Can you work these out from the model? Positions are in its coordinate system, mm. A direction names the side the tool comes from. Coordinates: 2 decimals unless noted, no trailing zeros. Order: outer loops, then holes, each group sorted by start corner. A loop starts at its lowest first (then second) coordinate and runs counter-clockwise, first axis right, second up. Notation, with made-up numbers: (53, 49.25) -> (111, 49.25) arc R9 ccw to (111, 62.25) -> close; hole circle Ø9 at (72, -22.75). An arc over 180 degrees is marked (long way). Answer in a Markdown table with one row per item. Add a question column.
1. We'd pull the mould along X, two halves only. Please class faces 1 (the face through (7.938, 0, 5)), 2 (the face through (6.49, 0.01, -12.21)), 3 (the face through (0, -0.794, -7)), 4 (the face through (14.288, 0, 0)): pulls with the +X half, pulls with the -X half, needs draft (parallel to the pull), parting line crosses it, or undercut.
2. Imagine slicing it at B-B on z = 12.7. Write out the boundary of the cut face in (x, y) (1 decimal), plus the area to 3 significant figures.
3. Imagine slicing it at D-D on x = -8.75. Write out the boundary of the cut face in (y, z), plus the area to 3 significant figures.
4. Imagine slicing it at A-A on z = -5. Write out the boundary of the cut face in (x, y).
5. Will these pins go through, and if not, where does the flat tip stop? pin 1 (6 mm diameter, centred on x = -7.94, z = -10.32, fed in from -Y); pin 2 (0.8 mm diameter, centred on x = -3.5, y = 0, fed in from +Z); pin 3 (4 mm diameter, centred on x = -12.5, z = 13.5, fed in from +Y); pin 4 (2.5 mm diameter, centred on x = -11.11, z = 12.7, fed in from +Y).
6. If I drill on line 1 along X through (y, z) = (-0.3, 12.7) (1 decimal); line 2 along X through (y, z) = (-0.3, 6.5); line 3 along X through (y, z) = (0, -12), over which ranges is the centre line in solid material (lowest first)? Write a range as [from, to].
7. On a 3-axis mill with a long thin cutter (end or side, diameter ignored), from which of +Z, -Z, +X, -X, +Y, -Y can I reach the whole of each face in a straight line? I mean faces 5 (the face through (0, 0, -5.556)), 6 (the face through (-10, 0, 11)), 7 (the face through (0, 0, -15.081)). Say none if no direction works.
8. Imagine slicing it at C-C on y = 0.4. Write out the boundary of the cut face in (x, z), plus the area to 3 significant figures.
from build123d import *

# Parameters (mm, degrees)
BOSS_EXTRUDE1_DEPTH = 0.79375
SKETCH2_W           = 6.35
SKETCH2_H           = 4.7625
CUT_EXTRUDE1_DEPTH  = 0.79375
SKETCH3_R           = 1.5875
SKETCH3_R_2         = 2.38125
CUT_EXTRUDE2_DEPTH  = 1.5875


with BuildPart() as part:
    # Sketch1 → Boss-Extrude1 (new, symmetric)
    with BuildSketch(Plane(origin=(0, 0, 0), x_dir=(1, 0, 0), z_dir=(0, 1, 0))):
        Polygon((14.2875, 15.08125), (-14.2875, 15.08125), (-14.2875, -15.08125), (-7.9375, -15.08125), (-7.9375, 5.55625), (7.9375, 5.55625), (7.9375, -15.08125), (14.2875, -15.08125), align=None)
    extrude(amount=BOSS_EXTRUDE1_DEPTH, both=True)

    # Sketch2 → Cut-Extrude1 (cut)
    with BuildSketch(Plane(origin=(0, 0.79375, 0), x_dir=(1, 0, 0), z_dir=(0, 1, 0))):
        with Locations((-11.1125, -12.7)):
            Rectangle(SKETCH2_W, SKETCH2_H)
        with Locations((11.1125, -12.7)):
            Rectangle(SKETCH2_W, SKETCH2_H)
    extrude(amount=-CUT_EXTRUDE1_DEPTH, mode=Mode.SUBTRACT)

    # Sketch3 → Cut-Extrude2 (cut)
    with BuildSketch(Plane(origin=(0, 0.79375, 0), x_dir=(1, 0, 0), z_dir=(0, 1, 0))):
        with Locations(Location((-11.1125, -12.7, 0), (0, 0, 270))):
            Circle(SKETCH3_R)
        with Locations(Location((-7.9375, 10.31875, 0), (0, 0, 270))):
            Circle(SKETCH3_R_2)
        with Locations(Location((11.1125, -12.7, 0), (0, 0, 270))):
            Circle(SKETCH3_R)
        with Locations(Location((7.9375, 10.31875, 0), (0, 0, 270))):
            Circle(SKETCH3_R_2)
    extrude(amount=-CUT_EXTRUDE2_DEPTH, mode=Mode.SUBTRACT)


solid = part.part
Answers follow:
| question | item | result |
|---|---|---|
| 1 | face 1 | undercut |
| 1 | face 2 | undercut |
| 1 | face 3 | needs draft |
| 1 | face 4 | pulls with the +X half |
| 2 | outline | (-14.3, -0.8) -> (-12.7, -0.8) -> (-12.7, 0) -> (-14.3, 0) -> close; (-9.5, -0.8) -> (-7.9, -0.8) -> (-7.9, 0) -> (-9.5, 0) -> close; (7.9, -0.8) -> (9.5, -0.8) -> (9.5, 0) -> (7.9, 0) -> close; (12.7, -0.8) -> (14.3, -0.8) -> (14.3, 0) -> (12.7, 0) -> close |
| 2 | area | 5.04 mm² |
| 3 | outline | (-0.79, -15.08) -> (0.79, -15.08) -> (0.79, -12.56) -> (-0.79, -12.56) -> close; (-0.79, -8.08) -> (0.79, -8.08) -> (0.79, 10.32) -> (0, 10.32) -> (0, 15.08) -> (-0.79, 15.08) -> close |
| 3 | area | 37.0 mm² |
| 4 | outline | (-14.29, -0.79) -> (-7.94, -0.79) -> (-7.94, 0.79) -> (-14.29, 0.79) -> close; (7.94, -0.79) -> (14.29, -0.79) -> (14.29, 0.79) -> (7.94, 0.79) -> close |
| 5 | pin 1 | stops at y = -0.79 |
| 5 | pin 2 | stops at z = -5.56 |
| 5 | pin 3 | stops at y = 0 |
| 5 | pin 4 | passes through |
| 6 | line 1 | x = [-14.3, -12.7], [-9.5, -7.9], [7.9, 9.5], [12.7, 14.3] |
| 6 | line 2 | x = [-14.29, -7.94], [7.94, 14.29] |
| 6 | line 3 | x = [-14.29, -9.62], [-6.25, 6.25], [9.62, 14.29] |
| 7 | face 5 | +Z, +Y, -Y |
| 7 | face 6 | +Z, +X, -X, +Y |
| 7 | face 7 | -Z, +X, -X, +Y, -Y |
| 8 | outline | (-14.29, -15.08) -> (14.29, -15.08) -> (14.29, 10.32) -> (7.94, 10.32) -> (7.94, -5.56) -> (-7.94, -5.56) -> (-7.94, 10.32) -> (-14.29, 10.32) -> close; hole circle Ø4.76 at (-7.94, -10.32); hole circle Ø4.76 at (7.94, -10.32) |
| 8 | area | 438 mm² |
